Here's how the part is built. I have some questions about the finished solid (model axes, mm). Face numbers are marked on the shaded views. A direction names the side the tool comes from. Coordinates: 2 decimals unless noted, no trailing zeros. Write each loop counter-clockwise with the first axis right and the second up, starting at its lowest first coordinate (ties: lowest second). Pieces come first, ordered by that corner, then holes. Notation, with made-up numbers: M 8,-29.5 L 24,-29.5 A20 cw 24,-0.5 Z; hole C 31,-36.5 d9. An arc over 180 degrees is marked long. Use a Markdown table: item, result.
Autodesk Fusion 360 part; units mm, degrees
sketch "Skizze1" plane through (0, 0, 0) normal (0, 0, 1) x (1, 0, 0)
  circle A0 centre (0, 0) radius 30.8
  dimension "d1" = 61.6
extrude "Extrusion1" add sketch "Skizze1" along normal blind 12
sketch "Skizze2" plane through (0, 0, 12) normal (0, 0, 1) x (-1, 0, 0)
  circle A0 centre (0, 0) radius 30.8
  circle A1 centre (0, 0) radius 40
  dimension "d4" = 80
extrude "Extrusion2" add sketch "Skizze2" along normal blind 3 contours A0 | A1
extrude "Extrusion4" add 1 faces at (6.9618, -9.4552, 0) along direction (0, 0, -1) blind 4
sketch "Skizze4" plane through (0, 0, -4) normal (0, 0, -1) x (1, 0, 0)
  circle A0 centre (0, 0) radius 30.8
  circle A1 centre (0, 0) radius 35
  dimension "d14" = 70
extrude "Extrusion5" add sketch "Skizze4" along normal blind 3 contours A0 | A1
chamfer "Fase3" distance 2 angle 45 1 edges at (-32.6315, 12.6565, -7)
chamfer "Fase5" distance 3 angle 45 1 edges at (37.2931, 14.4646, 15)
sketch "Skizze5" plane through (0, 0, 15) normal (0, 0, 1) x (-1, 0, 0)
  circle A0 centre (0, 0) radius 37
  circle A1 centre (0, 0) radius 27
  dimension "d20" = 54
chamfer "Fase7" distance 4 angle 45 1 edges at (-28.7157, 11.1378, -4)
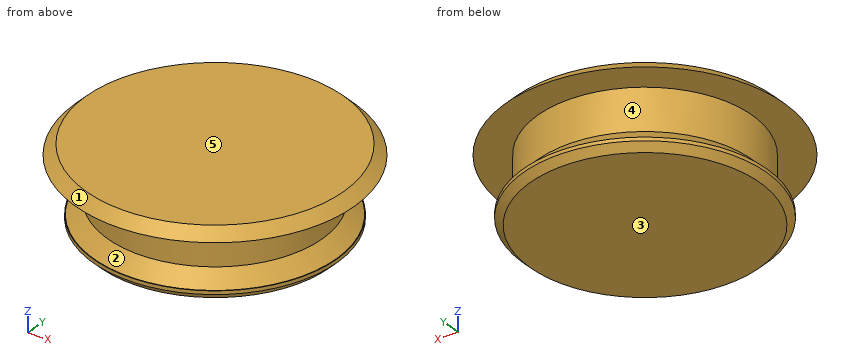
1. Suppose I cut it at C-C on z = -2.5. Write out the boundary of the cut face in (x, y), and give its area (3 significant figures).
Answers follow:
| item | result |
|---|---|
| outline | C 0,0 d66.6 |
| area | 3,480 mm2 |
2. Will these pins go through, and if not, where does the flat tip stop? pin 1 Ø5 at (x, z) = (23.5, 1) entering from +Y; pin 2 Ø10 at (y, z) = (-13.5, 0.5) entering from +X; pin 3 Ø2 at (y, z) = (27, 1.5) entering from +X.
Answers follow:
| item | result |
|---|---|
| pin 1 | stops at y = 22.96 |
| pin 2 | stops at x = 33.12 |
| pin 3 | stops at x = 16.51 |
3. We'd pull the mould along Z, two halves only. Please class the marked faces 3, 4 and 5: +Z half, -Z half, draft (parallel to the pull), parting line (faces both ways), or undercut.
Answers follow:
| item | result |
|---|---|
| face 3 | -Z half |
| face 4 | undercut |
| face 5 | +Z half |
4. Which directions (+Z, -Z, +X, -X, +Y, -Y) give clear straight access to the entire face, cutting with the end or side of a thin tool? Please do the marked faces 1 and 2.
Answers follow:
| item | result |
|---|---|
| face 1 | +Z |
| face 2 | none |
5. Suppose I cut it at D-D on z = 9. Write out the boundary of the cut face in (x, y), and give its area (3 significant figures).
Answers follow:
| item | result |
|---|---|
| outline | C 0,0 d61.6 |
| area | 2,980 mm2 |
6. I need wall thicknesses on probe 1 along Y at (x, z) = (-1, 10.25); probe 2 along Y at (x, z) = (-19, 1.5); probe 3 along X at (y, z) = (27, -1). Which ranges of each line are inside material? Lowest first, please.
Answers follow:
| item | result |
|---|---|
| probe 1 | y = -30.78 to 30.78 |
| probe 2 | y = -24.24 to 24.24 |
| probe 3 | x = -16.8 to 16.8 |
